The figure shows three views and two pictorial views of one solid part (mm, origin at its lowest corner). Answer the questions. A direction names the side the tool comes from. Round coordinates to 2 decimals unless told otherwise and drop trailing zeros. Write each loop counter-clockwise with the first axis right and the second up, starting at its lowest first coordinate (ties: lowest second). Pieces come first, ordered by that corner, then holes.
Item 1: A tool of negligible diameter and unlimited length cuts with its end or side. For the marked faces 1 and 2, from which of +Z, -Z, +X, -X, +Y, -Y can it reach the whole face along a straight path? Write none if from no direction.
Item 2: Find section C-C on x = 5.25. Give the vertices of the cut face in (y, z), then the cut area to 3 significant figures.
Item 3: Find the intervals of material crossed by probe 1 along Y at (x, z) = (1.7, 11); probe 2 along X at (y, z) = (16.5, 19.25); probe 3 along Y at (x, z) = (3.25, 7.75), in increasing order.
Item 4: Find section A-A on z = 11. Give the vertices of the cut face in (x, y).
Item 5: Each of these flat-tipped pins is pushed along its axis until it touches: pin 1 (2 mm diameter, centred on x = 1, z = 16, fed in from -Y); pin 2 (1.5 mm diameter, centred on x = 4, z = 12, fed in from +Y); pin 3 (1.5 mm diameter, centred on x = 1, z = 2.5, fed in from -Y); pin 4 (7 mm diameter, centred on y = 11, z = 11, fed in from +X). Where does it stop, or does it pass through?
Item 6: For a pull along Y with two mould halves and no side action, classify the marked faces 3, 4 and 5 as +Y half, -Y half, draft (parallel to the pull), parting line (faces both ways), or undercut.
Item 7: Find section D-D on y = 5.75. Give the vertices of the cut face in (x, z).
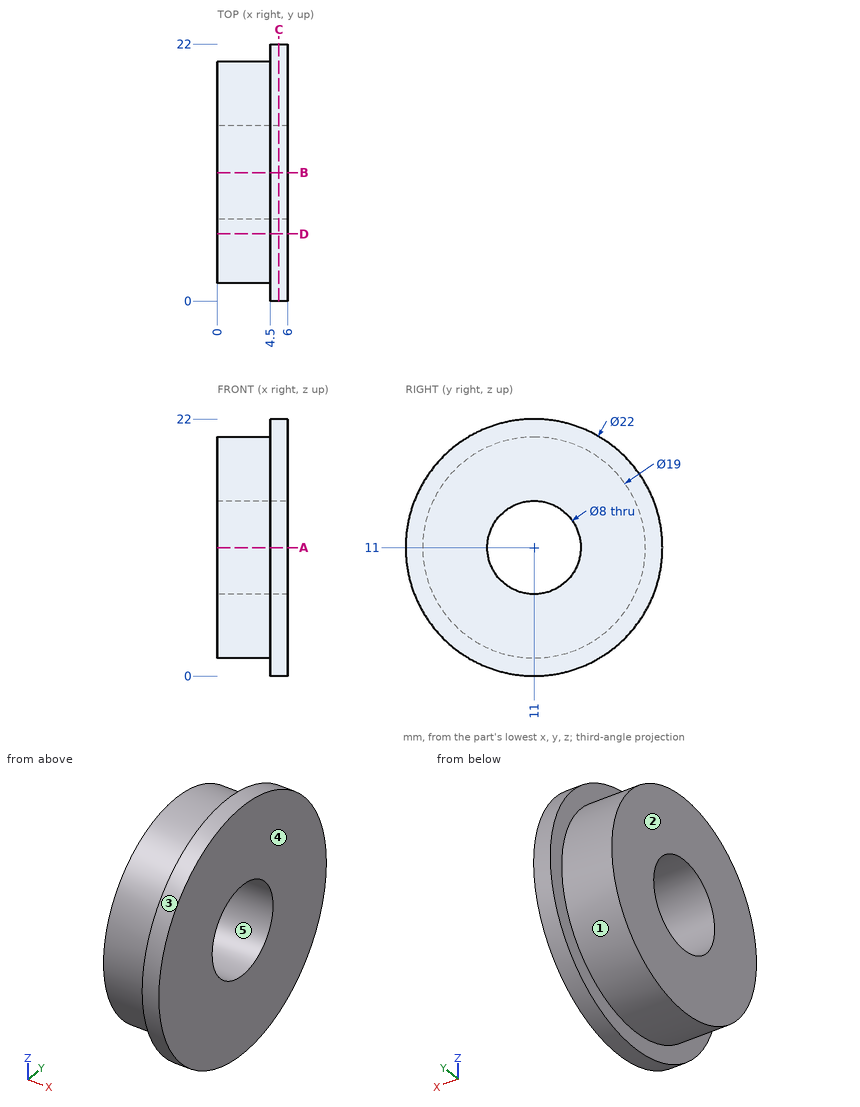
Check values:
1. face 1: -X
1. face 2: +Z, -Z, -X, +Y, -Y
2. outline: circle Ø22 at (11, 11); hole circle Ø8 at (11, 11)
2. area: 330 mm2
3. probe 1: y = 1.5 to 7, 15 to 20.5
3. probe 2: x = 4.5 to 6
3. probe 3: y = 2.07 to 8.67, 13.33 to 19.93
4. outline: (0, 1.5) - (4.5, 1.5) - (4.5, 0) - (6, 0) - (6, 7) - (0, 7) - close; (0, 15) - (6, 15) - (6, 22) - (4.5, 22) - (4.5, 20.5) - (0, 20.5) - close
5. pin 1: stops at y = 2.38
5. pin 2: stops at y = 21.99
5. pin 3: stops at y = 5.51
5. pin 4: passes through
6. face 3: parting line
6. face 4: draft
6. face 5: undercut
7. outline: (0, 3.08) - (4.5, 3.08) - (4.5, 1.33) - (6, 1.33) - (6, 20.67) - (4.5, 20.67) - (4.5, 18.92) - (0, 18.92) - close
